Read the model definition and answer for the solid it produces. Units are mm, in the model's axes. A direction names the side the tool comes from. Round coordinates to 2 decimals unless told otherwise and drop trailing zeros. Order: outer loops, then holes, each group sorted by start corner. A loop starts at its lowest first (then second) coordinate and runs counter-clockwise, first axis right, second up. Notation, with made-up numbers: (15, 62.5) -> (37, 62.5) arc R22 cw to (37, 98.5) -> close; hole circle Ø8 at (-5.5, 31). An arc over 180 degrees is marked (long way). One line per item, written item: value. Start each with the question number.
1. Section D-D (y = -10) is taken. Give the vertices of the cut face in (x, z) (3 decimals), then the cut area to 3 significant figures.
2. The mould has two halves that part along X. Classify faces 4 (the face through (6.85, 5.37, 0.11)), 5 (the face through (0, 0, -7.875)), 6 (the face through (-13, 0, -16.75)): released by +X, released by -X, zero draft, split by the parting line, or undercut.
3. Section A-A (y = 9) is taken. Give the vertices of the cut face in (x, z) (3 decimals), then the cut area to 3 significant figures.
4. For faces 1 (the face through (0, 0, 11.305)), 2 (the face through (0, 0, -11.305)), 3 (the face through (-5.127, 2.385, 0.11)), determine the directions among +Z, -Z, +X, -X, +Y, -Y from which every point of the face is accessible in a straight line to the end or side of a thin tool.
5. Section B-B (z = -12) is taken. Give the vertices of the cut face in (x, y).
6. Consider line 1 (Z direction, x = 22, y = -6.5) (3 decimals); line 2 (Z direction, x = -6.5, y = -2) (3 decimals); line 3 (X direction, y = 7, z = -3). Determine where each line is inside the solid, lowest interval first.
7. Flat-ended cylindrical pins translate along their axes: pin 1 Ø2 at (x, z) = (-3, 9) entering from -Y; pin 2 Ø6 at (x, z) = (0, -7.5) entering from +Y; pin 3 Ø10 at (x, z) = (6, -5) entering from -Y. Find the tip coordinate at first contact, or state that the pin passes through.
8. Section C-C (x = -12.7) is taken. Give the vertices of the cut face in (y, z) (3 decimals).
from build123d import *

# Parameters (mm, degrees)
SKETCH_2_R        = 7.94
EXTRUDE_1_DEPTH   = 7.875
EXTRUDE_1_2_DEPTH = 7.875
EXTRUDE_2_DEPTH   = 3.43
SKETCH_4_R        = 3.97
EXTRUDE_3_DEPTH   = 16.75
CHAMFER_1_SIZE    = 0.686


with BuildPart() as part:
    # Sketch 2 → Extrude 1 (new, symmetric)
    with BuildSketch(Plane.XY):
        with Locations((12.7, 0)):
            Circle(SKETCH_2_R)
    extrude(amount=EXTRUDE_1_DEPTH, both=True)



with BuildPart() as body_2:
    # Sketch 2 → Extrude 1 2 (new, symmetric)
    with BuildSketch(Plane.XY):
        with Locations((-12.7, 0)):
            Circle(SKETCH_2_R)
    extrude(amount=EXTRUDE_1_2_DEPTH, both=True)


with BuildPart() as part_1:
    add(part.part)

    add(body_2.part)  # Extrude 2 merges body 2
    # Sketch 3 → Extrude 2 (add)
    with BuildSketch(Plane.XY.offset(7.875)):
        with BuildLine():
            ThreePointArc((-10.428153415, 11.849174574), (-24.765, 0), (-10.428153415, -11.849174574))
            ThreePointArc((-10.428153415, -11.849174574), (0, -10.8585), (10.428153415, -11.849174574))
            ThreePointArc((10.428153415, -11.849174574), (24.765, 0), (10.428153415, 11.849174574))
            ThreePointArc((10.428153415, 11.849174574), (0, 10.8585), (-10.428153415, 11.849174574))
        make_face()
    extrude_2 = extrude(amount=EXTRUDE_2_DEPTH)

    # Mirror 1: Extrude 2 across plane
    add(extrude_2.mirror(Plane.XY))

    # Sketch 4 → Extrude 3 (add, symmetric)
    with BuildSketch(Plane.XY):
        with Locations((12.7, 0)):
            Circle(SKETCH_4_R)
        with Locations((-12.7, 0)):
            Circle(SKETCH_4_R)
    extrude(amount=EXTRUDE_3_DEPTH, both=True)

    # Chamfer 1
    chamfer_1_edges = [part_1.edges().sort_by_distance(p)[0] for p in [
        (8.73, 0, -16.75),
        (8.73, 0, 16.75),
        (-16.67, 0, -16.75),
        (-16.67, 0, 16.75),
    ]]
    chamfer(chamfer_1_edges, length=CHAMFER_1_SIZE)


solid = part_1.part
Answer:
1. outline: (-19.45, -11.305) -> (19.45, -11.305) -> (19.45, -7.875) -> (-19.45, -7.875) -> close; (-19.45, 7.875) -> (19.45, 7.875) -> (19.45, 11.305) -> (-19.45, 11.305) -> close
1. area: 267 mm^2
2. face 4: undercut
2. face 5: undercut
2. face 6: zero draft
3. outline: (-20.735, -11.305) -> (20.735, -11.305) -> (20.735, -7.875) -> (-20.735, -7.875) -> close; (-20.735, 7.875) -> (20.735, 7.875) -> (20.735, 11.305) -> (-20.735, 11.305) -> close
3. area: 284 mm^2
4. face 1: +Z
4. face 2: -Z
4. face 3: none
5. outline: circle Ø7.94 at (-12.7, 0); circle Ø7.94 at (12.7, 0)
6. line 1: -11.305 to -7.875, 7.875 to 11.305
6. line 2: -11.305 to 11.305
6. line 3: -16.45 to -8.95, 8.95 to 16.45
7. pin 1: y = -11
7. pin 2: y = 10.94
7. pin 3: y = -11.79
8. outline: (-12.065, -11.305) -> (-3.97, -11.305) -> (-3.97, -16.064) -> (-3.284, -16.75) -> (3.284, -16.75) -> (3.97, -16.064) -> (3.97, -11.305) -> (12.065, -11.305) -> (12.065, -7.875) -> (7.94, -7.875) -> (7.94, 7.875) -> (12.065, 7.875) -> (12.065, 11.305) -> (3.97, 11.305) -> (3.97, 16.064) -> (3.284, 16.75) -> (-3.284, 16.75) -> (-3.97, 16.064) -> (-3.97, 11.305) -> (-12.065, 11.305) -> (-12.065, 7.875) -> (-7.94, 7.875) -> (-7.94, -7.875) -> (-12.065, -7.875) -> close
